Check sheet for the modelled part. Datum: model origin and axes. Units: mm. Face numbers are marked on the shaded views. A direction names the side the tool comes from. Round coordinates to 2 decimals unless told otherwise and drop trailing zeros. Order: outer loops, then holes, each group sorted by start corner. A loop starts at its lowest first (then second) coordinate and runs counter-clockwise, first axis right, second up.
Q1. Mould release check, pull along X, two halves, no side actions. Record for the marked faces 3, 4 and 5: +X half, -X half, draft (parallel to the pull), parting line (faces both ways), or undercut.
Q2. Cross-section at B-B on z = 0. Record the cut outline in (x, y).
Q3. Set-up check for the marked faces 1 and 2: record each of +Z, -Z, +X, -X, +Y, -Y from which the full face is reachable in a straight line by a thin tool's end or side.
Q4. Cross-section at C-C on y = 3.9. Record the cut outline in (x, z), then the cut area to 3 significant figures.
Q5. Scan lines: probe 1 along X at (y, z) = (3.45, 0); probe 2 along Z at (x, y) = (0, 1.55). Record each from-to range of solid material in increasing order.
Q6. Cross-section at A-A on x = 0. Record the cut outline in (y, z), then the cut area to 4 significant figures.
Q7. Depth check by flat-ended pin: P1, Ø2, axis at x = 4, y = 2, coming from the -Z side; P2, Ø6, axis at x = 9, z = 8.5, coming from the -Y side; P3, Ø7, axis at x = 5.5, z = -3, coming from the +Y side; P4, Ø2, axis at x = 1.5, y = 1.5, coming from the +Z side. Enter the tip coordinate at first touch or a pass-through.
Q8. Cross-section at D-D on x = -12.5. Record the cut outline in (y, z).
Autodesk Inventor part; units mm, degrees
ref_plane "YZ Plane" through (0, 0, 0) normal (1, 0, 0) x (0, 1, 0)
ref_plane "XZ Plane" through (0, 0, 0) normal (0, 1, 0) x (-1, 0, 0)
ref_plane "XY Plane" through (0, 0, 0) normal (0, 0, 1) x (1, 0, 0)
sketch "Sketch1" plane through (0, 0, 0) normal (0, 1, 0) x (-1, 0, 0)
  circle A0 centre (0, 0) radius 15
  dimension "d0" = 30
extrude "Extrusion1" add sketch "Sketch1" along normal blind 2
sketch "Sketch2" plane through (0, 2, 0) normal (0, 1, 0) x (1, 0, 0)
  circle A0 centre (0, 0) radius 13
  dimension "d3" = 26
extrude "Extrusion2" add sketch "Sketch2" along normal blind 3.5
sketch "Sketch3" plane through (0, 5.5, 0) normal (0, 1, 0) x (1, 0, 0)
  circle A0 centre (0, 0) radius 11.25
  dimension "d6" = 22.5
extrude "Extrusion3" cut sketch "Sketch3" against normal blind 3.5
sketch "Sketch4" plane through (0, 2, 0) normal (0, 1, 0) x (1, 0, 0)
  circle A0 centre (0, 0) radius 4.25
  dimension "d9" = 8.5
extrude "Extrusion4" cut sketch "Sketch4" against normal through all
properties part number "poulie"
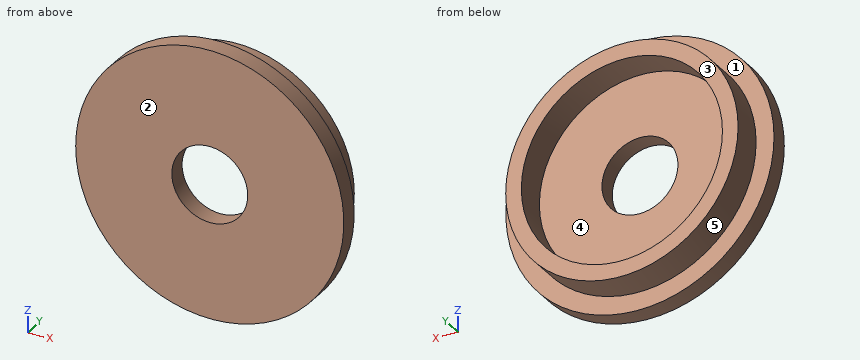
Results found:
1. face 3: draft
1. face 4: undercut
1. face 5: parting line
2. outline: (-15, 0) - (-4.25, 0) - (-4.25, 2) - (-11.25, 2) - (-11.25, 5.5) - (-13, 5.5) - (-13, 2) - (-15, 2) - close; (4.25, 0) - (15, 0) - (15, 2) - (13, 2) - (13, 5.5) - (11.25, 5.5) - (11.25, 2) - (4.25, 2) - close
3. face 1: +Y
3. face 2: +Z, -Z, +X, -X, -Y
4. outline: circle Ø26 at (0, 0); hole circle Ø22.5 at (0, 0)
4. area: 133 mm2
5. probe 1: x = -13 to -11.25, 11.25 to 13
5. probe 2: z = -15 to -4.25, 4.25 to 15
6. outline: (0, -15) - (2, -15) - (2, -13) - (5.5, -13) - (5.5, -11.25) - (2, -11.25) - (2, -4.25) - (0, -4.25) - close; (0, 4.25) - (2, 4.25) - (2, 11.25) - (5.5, 11.25) - (5.5, 13) - (2, 13) - (2, 15) - (0, 15) - close
6. area: 55.25 mm2
7. P1: stops at z = -14.7
7. P2: stops at y = 0
7. P3: stops at y = 2
7. P4: stops at z = 14.99
8. outline: (0, -8.29) - (2, -8.29) - (2, -3.57) - (5.5, -3.57) - (5.5, 3.57) - (2, 3.57) - (2, 8.29) - (0, 8.29) - close
